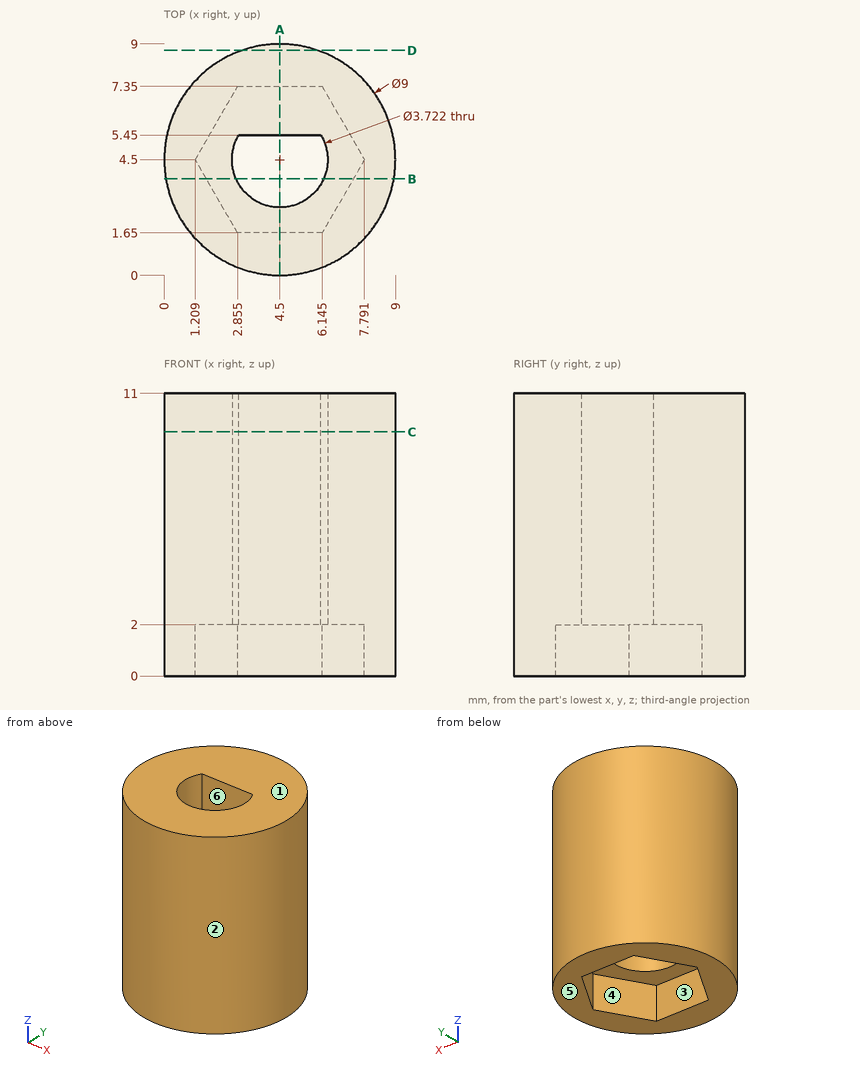
The drawing under review shows one solid part. Ordinate dimensions are in mm from its lowest x, y, z. A direction names the side the tool comes from. Give positions to 0.01 mm unless a question says otherwise; leave off trailing zeros. Loops run counter-clockwise (first coordinate to the right, second up) from the corner with the lowest first, then second, coordinate; pieces in that order, holes last. Notation, with made-up numbers: M 36,42.5 L 61,42.5 A16 cw 61,66.5 Z; hole C 78,48.5 d6. An arc over 180 degrees is marked long. One line per question, with ' | ' between items. Start each with the question number.
1. The part is to be moulded in two halves that separate along Y. For the marked faces 1, 2 and 3, say which applies: released by +Y, released by -Y, zero draft, split by the parting line, or undercut.
2. To check wall thickness, follow L1, parallel to Y at x = 4.5, z = 7.25; L2, parallel to Z at x = 4.25, y = 6.5; L3, parallel to X at y = 5.25, z = 7.75. State the ranges of each line that lie inside material, in increasing order.
3. For the marked faces 4, 5 and 6, list the 3-axis set-ups (+Z, -Z, +X, -X, +Y, -Y) from which the entire face can be reached by the end or side of a thin tool; tool diameter is ignored.
4. Add section B-B (y = 3.75). Write out the cut boundary in (x, z).
5. Add section D-D (y = 8.75). Write out the cut boundary in (x, z).
6. Add section A-A (x = 4.5). Write out the cut boundary in (y, z).
7. Insertion check: P1, Ø1.5, axis at x = 4, z = 9, coming from the +Y side; P2, Ø5, axis at x = 1, z = 2.5, coming from the -Y side; P3, Ø5, axis at x = 4.5, y = 4.5, coming from the -Z side; P4, Ø1, axis at x = 7, z = 3, coming from the -Y side. Each pin has a flat end and moves straight along its axis. Give the tip position at first contact, or say it passes through.
8. Add section C-C (z = 9.5). Write out the cut boundary in (x, y).
Worked out:
1) face 1: zero draft | face 2: split by the parting line | face 3: undercut
2) L1: y = 0 to 2.64, 5.45 to 9 | L2: z = 2 to 11 | L3: x = 0.06 to 2.8, 6.2 to 8.94
3) face 4: -Z | face 5: -Z, +X, -X, +Y, -Y | face 6: +Z, -Z
4) outline: M 0.06,0 L 1.64,0 L 1.64,2 L 2.8,2 L 2.8,11 L 0.06,11 Z; M 6.2,2 L 7.36,2 L 7.36,0 L 8.94,0 L 8.94,11 L 6.2,11 Z
5) outline: M 3.02,0 L 5.98,0 L 5.98,11 L 3.02,11 Z
6) outline: M 0,0 L 1.65,0 L 1.65,2 L 2.64,2 L 2.64,11 L 0,11 Z; M 5.45,2 L 7.35,2 L 7.35,0 L 9,0 L 9,11 L 5.45,11 Z
7) P1: stops at y = 9 | P2: stops at y = 0.11 | P3: stops at z = 2 | P4: stops at y = 0.47
8) outline: C 4.5,4.5 d9; hole M 2.9,5.45 A1.86 ccw long 6.1,5.45 Z
